```python
from build123d import *

# Parameters (mm, degrees)
F0_R          = 25.4
F1_DEPTH      = 25.4
F2_W          = 15.748
F2_H          = 5.08
F3_DEPTH      = 50.8
F3_DEPTH_BACK = 25.4


with BuildPart() as f1:
    # F0 (on Front) → F1 (new body)
    with BuildSketch(Plane.XZ):
        with Locations((-33.070799, 16.154399)):
            Circle(F0_R)
    extrude(amount=F1_DEPTH)

    # F2 (on Right) → F3 (join, two sides)
    with BuildSketch(Plane.YZ) as f3_sk:
        with Locations((-12.7, 31.060102)):
            Rectangle(F2_W, F2_H)
    extrude(amount=F3_DEPTH)
    extrude(f3_sk.sketch, amount=-F3_DEPTH_BACK)


solid = f1.part
```
Model file for the job. Use its own axes, mm. A direction names the side the tool comes from. Give positions to 0.01 mm unless a question says otherwise; leave off trailing zeros. Loops run counter-clockwise (first coordinate to the right, second up) from the corner with the lowest first, then second, coordinate; pieces in that order, holes last. Notation, with made-up numbers: (-10, -19) -> (33, -19) arc R18 ccw to (33, 5) -> close; hole circle Ø7 at (72.5, 66). An arc over 180 degrees is marked (long way). Use CSV: the item, a comma, the result in double quotes. Start each with the question number.
1) Slice it at C-C on y = -23.5. Give the cut face in (x, z), plus the area to 3 significant figures.
2) Mould opens along Y. For faces 1 (the flat face through (20, -13, 28.52)), 2 (the flat face through (19, -20.574, 31)), 3 (the flat face through (-33, 0, 17)) say: released by +Y, released by -Y, zero draft, split by the parting line, or undercut.
3) Slice it at B-B on y = -14. Give the cut face in (x, z).
4) Tool access for faces 4 (the flat face through (19, -13, 33.6)), 5 (the flat face through (-33, -25.4, 17)): list every direction of +Z, -Z, +X, -X, +Y, -Y with a clear straight run to the whole face (end or side of a thin tool).
5) Wall check: line 1 (Y direction, x = -10, z = 29); line 2 (Z direction, x = 41.5, y = -17); line 3 (Z direction, x = -32.5, y = -7). Give the ranges that are in metal, low to high.
6) Slice it at A-A on x = 6. Give the cut face in (y, z), plus the area to 3 significant figures.
7) Flat gauge pins, fed straight in: pin 1 Ø3 at (y, z) = (-18.5, 25.5) entering from -X; pin 2 Ø5 at (x, y) = (-15.5, -13.5) entering from -Z; pin 3 Ø10 at (y, z) = (-21, 22) entering from -X. Where does each tip first touch, or does it go through?
Computed values:
1,outline,"circle Ø50.8 at (-33.07, 16.15)"
1,area,"2,030 mm^2"
2,face 1,"zero draft"
2,face 2,"released by -Y"
2,face 3,"released by +Y"
3,outline,"(-14.61, 33.6) arc R25.4 ccw (long way) to (-10.88, 28.52) -> (50.8, 28.52) -> (50.8, 33.6) -> close"
4,face 4,"+Z, +X, +Y, -Y"
4,face 5,"+Z, -Z, +X, -X, -Y"
5,line 1,"y = -20.57 to -4.83"
5,line 2,"z = 28.52 to 33.6"
5,line 3,"z = -9.24 to 41.55"
6,outline,"(-20.57, 28.52) -> (-4.83, 28.52) -> (-4.83, 33.6) -> (-20.57, 33.6) -> close"
6,area,"80.0 mm^2"
7,pin 1,"stops at x = -57.23"
7,pin 2,"stops at z = -4.29"
7,pin 3,"stops at x = -58.46"
